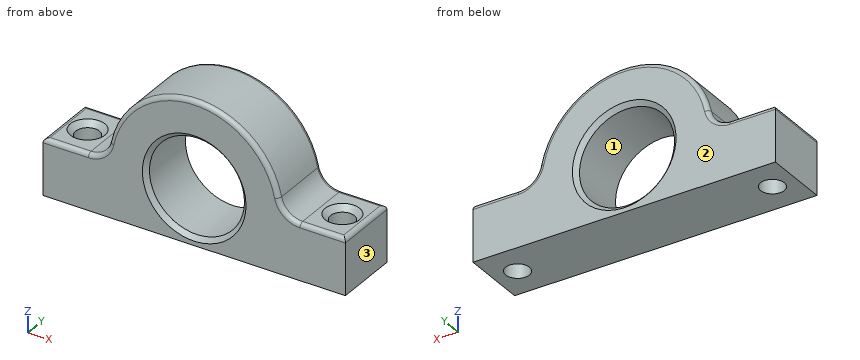
from build123d import *

# Parameters (mm, degrees)
F0_R           = 11
F1_DEPTH       = 15
F3_D           = 5.5
F3_CSINK_D     = 8
F3_CSINK_ANGLE = 90
F4_SIZE        = 1
F5_R           = 1


with BuildPart() as f1:
    # F0 (on Front) → F1 (new body)
    with BuildSketch(Plane.XZ):
        with BuildLine():
            ThreePointArc((24.494897, 0), (21.33262, 1.127017), (19.595918, 4))
            ThreePointArc((19.595918, 4), (0, 20), (-19.595918, 4))
            ThreePointArc((-19.595918, 4), (-21.33262, 1.127017), (-24.494897, 0))
            Line((-24.494897, 0), (-35, 0))
            Line((-35, 0), (-35, -13))
            Line((-35, -13), (35, -13))
            Line((35, -13), (35, 0))
            Line((35, 0), (24.494897, 0))
        make_face()
        Circle(F0_R, mode=Mode.SUBTRACT)
    extrude(amount=F1_DEPTH)

    # F3 (through all)
    with Locations(Plane.XY):
        with Locations((-29.494897, -7.5), (-29.494897, -22.5), (29.494897, -7.5), (29.494897, -22.5)):
            CounterSinkHole(F3_D / 2, F3_CSINK_D / 2, counter_sink_angle=F3_CSINK_ANGLE)

    # F4
    f4_edges = [f1.edges().sort_by_distance(p)[0] for p in [
        (-11, -15, 0),
        (-11, 0, 0),
    ]]
    chamfer(f4_edges, length=F4_SIZE)

    # F5
    f5_edges = [f1.edges().sort_by_distance(p)[0] for p in [
        (0, 0, 20),
        (0, -15, 20),
        (35, -7.5, 0),
        (-35, -7.5, 0),
    ]]
    fillet(f5_edges, radius=F5_R)


solid = f1.part
The model under review builds one solid part; all positions refer to its coordinate system, in mm. Face numbers are marked on the shaded views. Round coordinates to 2 decimals unless told otherwise and drop trailing zeros. Write each loop counter-clockwise with the first axis right and the second up, starting at its lowest first coordinate (ties: lowest second). Pieces come first, ordered by that corner, then holes. Notation, with made-up numbers: M 54.25,74.5 L 88.25,74.5 A27 ccw 88.25,100.5 Z; hole C -13.75,-31 d2. An arc over 180 degrees is marked long. Use a Markdown table: item, result. Add a question column.
Q1. Insertion check: pin 1 (7 mm diameter, centred on x = -29.49, y = -7.5, fed in from +Z); pin 2 (6 mm diameter, centred on x = 15, y = -3, fed in from +Z); pin 3 (7.5 mm diameter, centred on x = -30.5, y = -8, fed in from +Z). Each pin has a flat end and moves straight along its axis. Give the tip position at first contact, or say it passes through.
Q2. We need section A-A, the plane y = -7.5. State the section outline as (x, z) points.
Q3. We need section B-B, the plane x = 0. State the section outline as (y, z) points.
Q4. The part is to be moulded in two halves that separate along X. For the marked faces 1, 2 and 3, say which applies: pulls with the +X half, pulls with the -X half, needs draft (parallel to the pull), parting line crosses it, or undercut.
Q5. To check wall thickness, follow line 1 (X direction, y = -7.5, z = -6.25); line 2 (X direction, y = -7.5, z = -10); line 3 (X direction, y = -5.75, z = -12). State the ranges of each line that lie inside material, in increasing order.
Findings below:
| question | item | result |
|---|---|---|
| 1 | pin 1 | stops at z = -0.5 |
| 1 | pin 2 | stops at z = 16 |
| 1 | pin 3 | stops at z = 0 |
| 2 | outline | M -35,-13 L -32.24,-13 L -32.24,-1.25 L -33.49,0 L -34,0 A1 ccw -35,-1 Z; M -26.74,-13 L 26.74,-13 L 26.74,-1.25 L 25.49,0 L 24.49,0 A5 cw 19.6,4 A20 ccw -19.6,4 A5 cw -24.49,0 L -25.49,0 L -26.74,-1.25 Z; M 32.24,-13 L 35,-13 L 35,-1 A1 ccw 34,0 L 33.49,0 L 32.24,-1.25 Z; hole C 0,0 d22 |
| 3 | outline | M -15,-13 L 0,-13 L 0,-12 L -1,-11 L -14,-11 L -15,-12 Z; M -15,12 L -14,11 L -1,11 L 0,12 L 0,19 A1 ccw -1,20 L -14,20 A1 ccw -15,19 Z |
| 4 | face 1 | undercut |
| 4 | face 2 | needs draft |
| 4 | face 3 | pulls with the +X half |
| 5 | line 1 | x = -35 to -32.24, -26.74 to -9.05, 9.05 to 26.74, 32.24 to 35 |
| 5 | line 2 | x = -35 to -32.24, -26.74 to -4.58, 4.58 to 26.74, 32.24 to 35 |
| 5 | line 3 | x = -35 to -31.62, -27.37 to 27.37, 31.62 to 35 |
